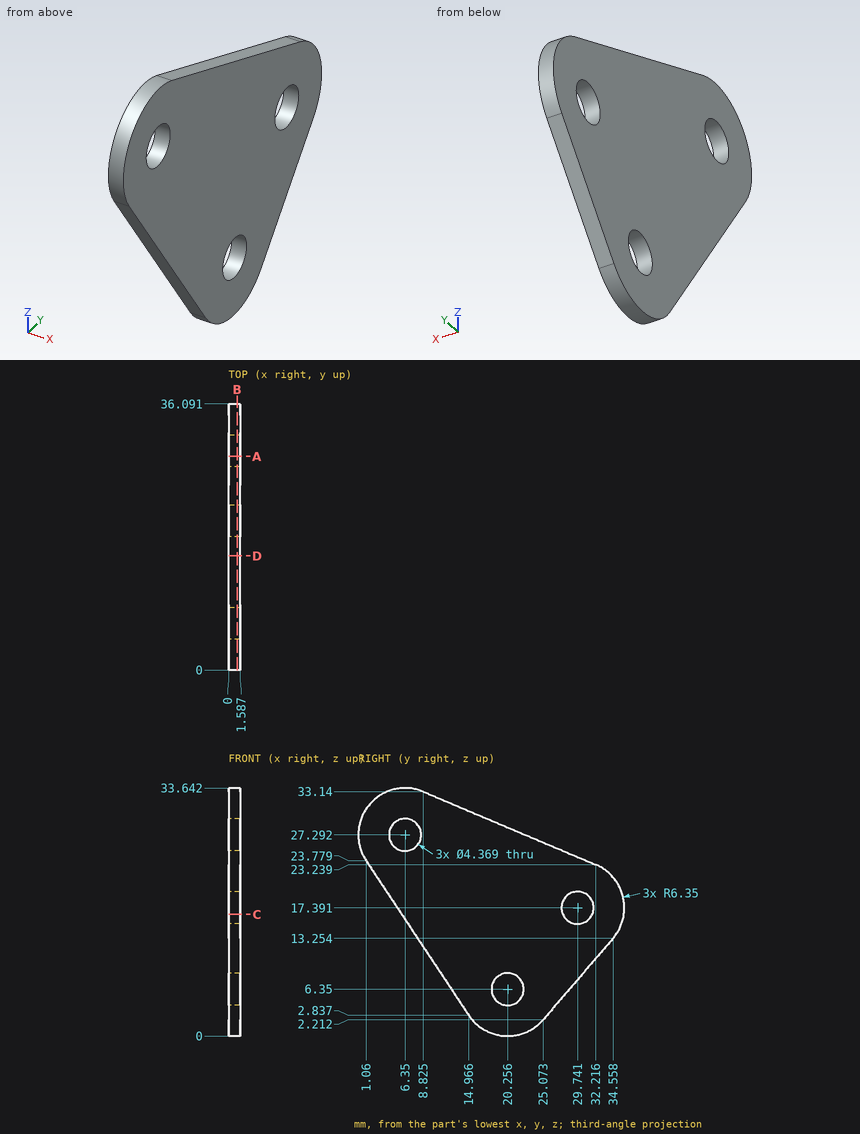
Answer from the drawing. Dimensions are ordinates in mm from the lowest x, y and z of the part. Give positions to 0.01 mm unless a question says otherwise; leave off trailing zeros. Loops run counter-clockwise (first coordinate to the right, second up) from the corner with the lowest first, then second, coordinate; pieces in that order, holes last. Notation, with made-up numbers: (-31.75, 12.25) -> (-5.75, 12.25) arc R26 ccw to (-5.75, 27.25) -> close; hole circle Ø1 at (-27, 43.5). An arc over 180 degrees is marked (long way). One line per question, with ' | ' between items. Start each with the question number.
1) Section C-C, the plane z = 16.5 is taken. Determine the outline of the cut face in (x, y) (1 decimal).
2) Section D-D, the plane y = 15.5 is taken. Determine the outline of the cut face in (x, z) (1 decimal).
3) Each of these flat-tipped pins is pushed along its axis until it touches: pin 1 (5 mm diameter, centred on y = 6.35, z = 27.29, fed in from -X); pin 2 (3.5 mm diameter, centred on y = 20.26, z = 6.35, fed in from +X). Where does it stop, or does it pass through?
4) Section A-A, the plane y = 29 is taken. Determine the outline of the cut face in (x, z).
5) Straight lines are drawn through the part: L1, parallel to Z at x = 0.15, y = 21 (1 decimal); L2, parallel to Y at x = 0.95, z = 29 (1 decimal); L3, parallel to Y at x = 1.05, z = 14 (1 decimal). For each, find the intervals that lie inside material, in ascending order.
6) Section B-B, the plane x = 1.15 is taken. State how many separate pieces and enclosed holes the cut face has, then the cut area to 3 significant figures.
Resolved:
1) outline: (0, 5.9) -> (1.6, 5.9) -> (1.6, 27.7) -> (0, 27.7) -> close; (0, 31.7) -> (1.6, 31.7) -> (1.6, 36) -> (0, 36) -> close
2) outline: (0, 2.1) -> (1.6, 2.1) -> (1.6, 30.3) -> (0, 30.3) -> close
3) pin 1: x = 0 | pin 2: through
4) outline: (0, 6.78) -> (1.59, 6.78) -> (1.59, 15.34) -> (0, 15.34) -> close; (0, 19.45) -> (1.59, 19.45) -> (1.59, 24.6) -> (0, 24.6) -> close
5) L1: 0 to 4.3, 8.4 to 28 | L2: 0.2 to 5, 7.7 to 18.6 | L3: 7.6 to 35.1
6) separate pieces: 1 | enclosed holes: 3 | area: 671 mm2
